Could you check a few things on this model? Use its own coordinates, in mm. Coordinates: 2 decimals unless noted, no trailing zeros. Loops run counter-clockwise (first coordinate to the right, second up) from the corner with the lowest first, then second, coordinate; pieces in that order, holes last. Notation, with made-up numbers: (39, 12.25) -> (50, 12.25) arc R20 cw to (50, 40.25) -> close; hole circle Ø10 at (-21.75, 87.25). An arc over 180 degrees is marked (long way). One line per question, with ' | ' between items.
Autodesk Fusion 360 part; units mm, degrees
sketch "Sketch1" plane through (0, 0, 0) normal (0, 1, 0) x (1, 0, 0)
  circle A0 centre (0, 0) radius 49
  circle A1 centre (0, 0) radius 51
  dimension "d1" = 98
  dimension "d4" = 102
extrude "Extrude2" add sketch "Sketch1" along normal blind 526
hole "Hole1" at (0, 6.1335, 51) direction (0, 0, -1) diameter 4 depth 2.0394 tip angle 180
mirror "Mirror1" about plane through (0, 0, 0) normal (0, 0, 1) of "Hole1"
1) If we section it at B-B on x = 30.5: Please give me the cut outline in (y, z).
Data:
outline: (0, -40.87) -> (526, -40.87) -> (526, -38.35) -> (0, -38.35) -> close; (0, 38.35) -> (526, 38.35) -> (526, 40.87) -> (0, 40.87) -> close
2) We'd pull the mould along X, two halves only. Please class faces 1 (the face through (26.34, 259.32, 41.32)), 2 (the face through (-11.056, 259.318, -49.787)), 3 (the face through (-19, 0, -46)): pulls with the +X half, pulls with the -X half, needs draft (parallel to the pull), parting line crosses it, or undercut.
Data:
face 1: undercut | face 2: parting line crosses it | face 3: needs draft
3) If we section it at C-C on y = 325: Please give me the cut outline in (x, z).
Data:
outline: circle Ø102 at (0, 0); hole circle Ø98 at (0, 0)
4) I need wall thicknesses on line 1 along Z through (x, y) = (1.5, 223); line 2 along X through (y, z) = (187, 0); line 3 along X through (y, z) = (404.5, 41). Which ranges of each line are inside material? Lowest first, please. Write a range as from..to.
Data:
line 1: -50.98..-48.98, 48.98..50.98 | line 2: -51..-49, 49..51 | line 3: -30.33..-26.83, 26.83..30.33
5) If we section it at A-A on z = 0: Please give me the cut outline in (x, y).
Data:
outline: (-51, 0) -> (-49, 0) -> (-49, 526) -> (-51, 526) -> close; (49, 0) -> (51, 0) -> (51, 526) -> (49, 526) -> close
6) I'm going to push flat-ended pins straight in: pin 1 Ø3 at (y, z) = (450, -10) entering from -X; pin 2 Ø4.5 at (x, y) = (0, 6.13) entering from +Z; pin 3 Ø3 at (x, z) = (-22, -40) entering from -Y; pin 4 Ø10 at (y, z) = (410, 18) entering from +X. Where does each tip first touch, or does it pass through?
Data:
pin 1: x = -50.29 | pin 2: z = 51 | pin 3: through | pin 4: x = 49.32
